Study the drawing (mm; zero at the part's minimum x, y, z) and answer. A direction names the side the tool comes from. Give positions to 0.01 mm unless a question says otherwise; leave off trailing zeros. Write each loop counter-clockwise with the first axis right and the second up, starting at its lowest first coordinate (ties: lowest second). Pieces come first, ordered by that corner, then holes. Notation, with made-up numbers: (27.25, -23.5) - (60.25, -23.5) arc R26 cw to (60.25, 12.5) - close; hole circle Ø8 at (53.5, 54). An arc over 180 degrees is marked (long way). One line per item, written item: value. Start each with the question number.
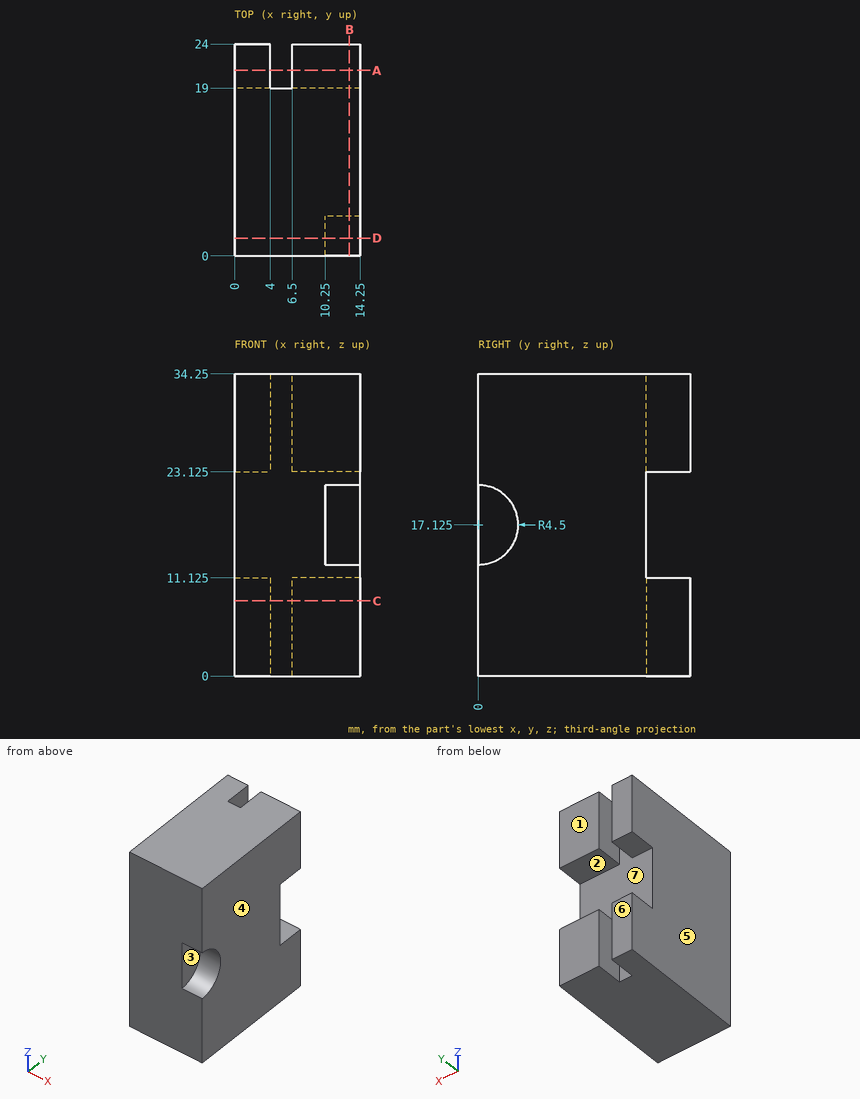
Item 1: Find section C-C on z = 8.5. Determine the outline of the cut face in (x, y), plus the area to 4 significant figures.
Item 2: The mould has two halves that part along X. Classify the marked faces 4, 5, 6 and 7: +X half, -X half, draft (parallel to the pull), parting line (faces both ways), or undercut.
Item 3: Find section A-A on y = 21. Determine the outline of the cut face in (x, z) (3 decimals).
Item 4: Find section B-B on x = 13. Determine the outline of the cut face in (y, z) (3 decimals).
Item 5: For the marked faces 1, 2 and 3, determine the directions among +Z, -Z, +X, -X, +Y, -Y from which every point of the face is accessible in a straight line to the end or side of a thin tool.
Item 6: Straight lines are drawn through the part: line 1 along Z through (x, y) = (9.5, 22.5) (3 decimals); line 2 along Y through (x, z) = (0.75, 15); line 3 along Y through (x, z) = (13.5, 20.5). For each, find the intervals that lie inside material, in ascending order.
Item 7: Find section D-D on y = 2. Determine the outline of the cut face in (x, z), plus the area to 3 significant figures.
Values:
1. outline: (0, 0) - (14.25, 0) - (14.25, 24) - (6.5, 24) - (6.5, 19) - (4, 19) - (4, 24) - (0, 24) - close
1. area: 329.5 mm^2
2. face 4: +X half
2. face 5: -X half
2. face 6: draft
2. face 7: undercut
3. outline: (0, 0) - (4, 0) - (4, 11.125) - (0, 11.125) - close; (0, 23.125) - (4, 23.125) - (4, 34.25) - (0, 34.25) - close; (6.5, 0) - (14.25, 0) - (14.25, 11.125) - (6.5, 11.125) - close; (6.5, 23.125) - (14.25, 23.125) - (14.25, 34.25) - (6.5, 34.25) - close
4. outline: (0, 0) - (24, 0) - (24, 11.125) - (19, 11.125) - (19, 23.125) - (24, 23.125) - (24, 34.25) - (0, 34.25) - (0, 21.625) arc R4.5 cw to (0, 12.625) - close
5. face 1: +Z, -Z, +X, -X, +Y
5. face 2: +X, -X, +Y
5. face 3: +X, -Y
6. line 1: 0 to 11.125, 23.125 to 34.25
6. line 2: 0 to 19
6. line 3: 2.98 to 19
7. outline: (0, 0) - (14.25, 0) - (14.25, 13.09) - (10.25, 13.09) - (10.25, 21.16) - (14.25, 21.16) - (14.25, 34.25) - (0, 34.25) - close
7. area: 456 mm^2
